Autodesk Inventor part; units mm, degrees
ref_plane "РабПлоскость1" through (0, -17.25, 7.5) normal (0, 0, 1) x (0, 1, 0)
ref_plane "YZ Plane" through (0, 0, 0) normal (1, 0, 0) x (0, 1, 0)
ref_plane "XZ Plane" through (0, 0, 0) normal (0, 1, 0) x (-1, 0, 0)
ref_plane "РабПлоскость1" through (0, -17.25, 7.5) normal (0, 0, 1) x (0, 1, 0)
sketch "Эскиз1" plane through (0, -17.25, 7.5) normal (0, 0, 1) x (0, 1, 0)
  line L0 (17.25, 0) -> (-17.1875, 0) construction
  line L1 (17.25, 10.35) -> (17.25, -10.35) construction
  line L2 (22.25, 12.85) -> (14.25, 12.85)
  line L3 (12.25, 10.85) -> (12.25, -10.85)
  line L4 (14.25, -12.85) -> (22.25, -12.85)
  line L5 (24.25, -10.85) -> (24.25, 10.85)
  line L6 (14.75, -12.85) -> (-9.95, -12.85) construction
  arc A0 (24.25, 10.85) -> (22.25, 12.85) centre (22.25, 10.85) ccw
  arc A1 (22.25, -12.85) -> (24.25, -10.85) centre (22.25, -10.85) ccw
  arc A2 (12.25, -10.85) -> (14.25, -12.85) centre (14.25, -10.85) ccw
  arc A3 (14.25, 12.85) -> (12.25, 10.85) centre (14.25, 10.85) ccw
  point P0 (12.25, -12.85)
  point P1 (12.25, 12.85)
  point P2 (24.25, -12.85)
  dimension "d1" = 5
  dimension "d2" = 12
  dimension "d3" = 2
  dimension "d6" = 2
extrude "Выдавливание1" add sketch "Эскиз1" along normal blind 4
sketch "Эскиз2" plane through (0, -17.25, 7.5) normal (0, 0, -1) x (-1, 0, 0)
  line L0 (10.35, 17.25) -> (-10.35, 17.25) construction
  line L1 (-10.85, 24.25) -> (10.85, 24.25) construction
  line L2 (-12.85, 14.25) -> (-12.85, 22.25)
  arc A0 (-12.85, 14.25) -> (-10.85, 12.25) centre (-10.85, 14.25) ccw
  line L3 (10.85, 12.25) -> (-10.85, 12.25) construction
  arc A1 (10.85, 12.25) -> (12.85, 14.25) centre (10.85, 14.25) ccw
  line L4 (12.85, 22.25) -> (12.85, 14.25)
  arc A2 (12.85, 22.25) -> (10.85, 24.25) centre (10.85, 22.25) ccw
  line L5 (-10.85, 24.25) -> (10.85, 24.25)
  arc A3 (-10.85, 24.25) -> (-12.85, 22.25) centre (-10.85, 22.25) ccw
  line L6 (12.85, 17.25) -> (-12.85, 17.25)
  point P0 (0, 17.25)
  point P1 (0, 17.25)
extrude "Выдавливание2" add sketch "Эскиз2" along normal blind 6
fillet "Сопряжение1" radius 2 2 edges at (-12.85, 0, 4.5) (12.85, 0, 4.5)
sketch "Эскиз3" plane through (0, -17.25, 1.5) normal (0, 0, -1) x (-1, 0, 0)
  arc A0 (-12.85, 19.25) -> (-10.85, 17.25) centre (-10.85, 19.25) ccw construction
  line L0 (-10.85, 17.25) -> (10.85, 17.25) construction
  arc A1 (10.85, 17.25) -> (12.85, 19.25) centre (10.85, 19.25) ccw construction
  line L1 (12.85, 19.25) -> (12.85, 22.25) construction
  arc A2 (12.85, 22.25) -> (10.85, 24.25) centre (10.85, 22.25) ccw construction
  line L2 (10.85, 24.25) -> (-10.85, 24.25) construction
  arc A3 (-10.85, 24.25) -> (-12.85, 22.25) centre (-10.85, 22.25) ccw construction
  line L3 (-12.85, 22.25) -> (-12.85, 19.25) construction
  line L4 (12.85, 20.75) -> (-12.85, 20.75) construction
  line L5 (0, 17.25) -> (0, 28) construction
  point P0 (10.5, 20.75)
  point P1 (-10.5, 20.75)
  dimension "d10" = 21
hole "Отверстие1" at (-10.5, 3.5, 1.5) at (10.5, 3.5, 1.5) direction (0, 0, 1) diameter 2.5 depth 4
chamfer "Фаска1" distance 0.2 angle 45 2 edges at (10.5, 2.25, 1.5) (-10.5, 2.25, 1.5)
sketch "Эскиз4" plane through (0, -17.25, 11.5) normal (0, 0, 1) x (1, 0, 0)
  line L0 (0, 17.25) -> (0, -22) construction
  line L1 (-10.85, 12.25) -> (10.85, 12.25) construction
  line L2 (-10.85, 12.25) -> (10.85, 12.25)
  line L3 (3, 12.25) -> (-3, 12.25)
  line L4 (-3, 12.25) -> (-3, -2.75)
  line L5 (-3, -2.75) -> (3, -2.75)
  line L6 (3, -2.75) -> (3, 12.25)
  dimension "d21" = 15
  dimension "d22" = 6
extrude "Выдавливание3" add sketch "Эскиз4" against normal blind 2
chamfer "Фаска2" distance 2 angle 45 2 edges at (-3, -5, 10.5) (3, -5, 10.5)
sketch "Эскиз5" plane through (0, -17.25, 11.5) normal (0, 0, 1) x (1, 0, 0)
  circle A0 centre (-10.5, 20.75) radius 1.45
  circle A1 centre (10.5, 20.75) radius 1.45
  circle A2 centre (-10.5, 20.75) radius 1.25
  point P0 (0, 17.25)
hole "Отверстие2" at (10.5, 3.5, 11.5) at (-10.5, 3.5, 11.5) direction (0, 0, -1) diameter 2.5 depth 4
chamfer "Фаска3" distance 0.3 angle 45 2 edges at (10.5, 4.75, 11.5) (-10.5, 4.75, 11.5)
properties part number "Кронштейн МК"
Part model, mm, in its own coordinate system. A direction names the side the tool comes from. Round coordinates to 2 decimals unless told otherwise and drop trailing zeros. Write each loop counter-clockwise with the first axis right and the second up, starting at its lowest first coordinate (ties: lowest second). Pieces come first, ordered by that corner, then holes. Notation, with made-up numbers: M 63.25,-29.75 L 68.25,-29.75 A18 ccw 68.25,-11.75 Z; hole C 85,68.25 d11. An arc over 180 degrees is marked long. One line per question, with ' | ' between items.
(1) Saw through at B-B on x = 10.5. Write the cut outline in (y, z).
Answer key:
outline: M -5,7.5 L 0,7.5 L 0,1.5 L 2.05,1.5 L 2.25,1.7 L 2.25,5.5 L 4.75,5.5 L 4.75,1.7 L 4.95,1.5 L 7,1.5 L 7,11.5 L 5.05,11.5 L 4.75,11.2 L 4.75,7.5 L 2.25,7.5 L 2.25,11.2 L 1.95,11.5 L -5,11.5 Z
(2) Pin check, flat tips, straight feed: pin 1 (0.8 mm diameter, centred on x = -10.5, y = 3.5, fed in from -Z); pin 2 (1.6 mm diameter, centred on y = -15, z = 11, fed in from -X); pin 3 (1.5 mm diameter, centred on x = -10.5, y = 3.5, fed in from +Z); pin 4 (8 mm diameter, centred on x = 7.5, y = -12.5, fed in from -Z). Stop position of each tip, or through.
Answer key:
pin 1: stops at z = 5.5 | pin 2: stops at x = -3 | pin 3: stops at z = 7.5 | pin 4: passes through
(3) Saw through at C-C on y = 3.5. Write the cut outline in (x, z), then the cut area to 3 significant figures.
Answer key:
outline: M -12.85,1.5 L -11.95,1.5 L -11.75,1.7 L -11.75,5.5 L -9.25,5.5 L -9.25,1.7 L -9.05,1.5 L 9.05,1.5 L 9.25,1.7 L 9.25,5.5 L 11.75,5.5 L 11.75,1.7 L 11.95,1.5 L 12.85,1.5 L 12.85,11.5 L 12.05,11.5 L 11.75,11.2 L 11.75,7.5 L 9.25,7.5 L 9.25,11.2 L 8.95,11.5 L -8.95,11.5 L -9.25,11.2 L -9.25,7.5 L -11.75,7.5 L -11.75,11.2 L -12.05,11.5 L -12.85,11.5 Z | area: 217 mm^2
(4) Saw through at A-A on z = 3. Write the cut outline in (x, y), then the cut area to 3 significant figures.
Answer key:
outline: M -12.85,2 A2 ccw -10.85,0 L 10.85,0 A2 ccw 12.85,2 L 12.85,5 A2 ccw 10.85,7 L -10.85,7 A2 ccw -12.85,5 Z; hole C -10.5,3.5 d2.5; hole C 10.5,3.5 d2.5 | area: 167 mm^2
(5) 3-axis set-ups, long thin cutter, end or side, ignore diameter. For faces 1 (the face through (3, -14, 11)), 2 (the face through (0, 0, 5)), 3 (the face through (0, -5, 9)): which of +Z, -Z, +X, -X, +Y, -Y reach the whole face in a straight line?
Answer key:
face 1: +Z, -Z, +X, -Y | face 2: -Z, +X, -X, -Y | face 3: -Z, -Y
(6) Saw through at D-D on z = 6.25. Write the cut outline in (x, y), then the cut area to 3 significant figures.
Answer key:
outline: M -12.85,2 A2 ccw -10.85,0 L 10.85,0 A2 ccw 12.85,2 L 12.85,5 A2 ccw 10.85,7 L -10.85,7 A2 ccw -12.85,5 Z | area: 176 mm^2
(7) Two-plate mould, pull along X, no slides. Class faces 4 (the face through (0, -20, 11)), 5 (the face through (-11, 3, 5.5)), 6 (the face through (12.85, 2, 8)), 7 (the face through (-12.25, -4.43, 9.47)): released by +X, released by -X, zero draft, split by the parting line, or undercut.
Answer key:
face 4: zero draft | face 5: undercut | face 6: released by +X | face 7: released by -X
(8) Probe line 1 along X through (y, z) = (3.5, 3.4); line 2 along Y through (x, z) = (-10.5, 2.6); line 3 along Y through (x, z) = (10.5, 10.15). List the from-to ranges inside material, lowest first.
Answer key:
line 1: x = -12.85 to -11.75, -9.25 to 9.25, 11.75 to 12.85 | line 2: y = 0 to 2.25, 4.75 to 7 | line 3: y = -5 to 2.25, 4.75 to 7
